Verification items for the finished model (mm, model axes). Face numbers are marked on the shaded views. A direction names the side the tool comes from. Round coordinates to 2 decimals unless told otherwise and drop trailing zeros. Order: outer loops, then holes, each group sorted by start corner. A loop starts at its lowest first (then second) coordinate and runs counter-clockwise, first axis right, second up. Notation, with made-up numbers: M -10.5,17 L 35.5,17 A15 ccw 35.5,24 Z; hole C -11,78 d9. An arc over 180 degrees is marked long. One line per item, written item: value. Start each with the question number.
from build123d import *

# Parameters (mm, degrees)
F0_W     = 63.5000000107
F0_H     = 19.05
F1_DEPTH = 63.5
F0_W_2   = 19.0499999893
F2_DEPTH = 25.4
F3_DEPTH = 15.875
F0_W_3   = 25.4
F0_H_2   = 19.0499999893
F5_R     = 6.35


with BuildPart() as f1:
    # F0 (on Front) → F1 (new body, symmetric)
    with BuildSketch(Plane.XZ):
        with Locations((-9.5249999946, 0)):
            Rectangle(F0_W, F0_H)
    extrude(amount=F1_DEPTH, both=True)

    # F0 (on Front) → F2 (join, symmetric)
    with BuildSketch(Plane.XZ):
        with Locations((31.7500000054, 0)):
            Rectangle(F0_W_2, F0_H)
        with BuildLine():
            Line((22.2250000107, 9.525), (41.275, 9.525))
            Line((41.275, 9.525), (41.275, 27.0002))
            ThreePointArc((41.275, 27.0002), (45.9246798487, 38.2255201513), (57.15, 42.8752))
            Line((57.15, 42.8752), (60.325, 42.8752))
            Line((60.325, 42.8752), (60.325, 61.9251999893))
            Line((60.325, 61.9251999893), (57.1730846286, 61.9251999893))
            Line((57.1730846286, 61.9251999893), (57.15, 61.9251999893))
            ThreePointArc((57.15, 61.9251999893), (32.4542956746, 51.6959043254), (22.2250000107, 27.0002))
            Line((22.2250000107, 27.0002), (22.2250000107, 9.525))
        make_face()
    extrude(amount=F2_DEPTH, both=True)

    # F0 (on Front) → F3 (join)
    with BuildSketch(Plane.XZ):
        with BuildLine():
            Line((-41.275, 9.525), (22.2250000107, 9.525))
            Line((22.2250000107, 9.525), (22.2250000107, 27.0002))
            ThreePointArc((22.2250000107, 27.0002), (32.4542956746, 51.6959043254), (57.15, 61.9251999893))
            add(Edge.make_bspline(
                [(-41.275, 9.525), (-41.275, 48.5757485088), (19.736442486, 61.9251999893), (57.15, 61.9251999893)],
                knots=[0, 0, 0, 0, 111.5045361585, 111.5045361585, 111.5045361585, 111.5045361585], degree=3))
        make_face()
    extrude(amount=F3_DEPTH)

    # F0 (on Front) → F4 (revolve)
    with BuildSketch(Plane.XZ):
        with Locations((73.025, 52.4001999946)):
            Rectangle(F0_W_3, F0_H_2)
    revolve(axis=Axis((60.325, 0, 52.3875), (0, 0, 1)))

    # F5
    f5_edges = [f1.edges().sort_by_distance(p)[0] for p in [
        (-41.275, -63.5, 0),
        (22.225, -63.5, 0),
        (-41.275, 63.5, 0),
        (22.225, 63.5, 0),
    ]]
    fillet(f5_edges, radius=F5_R)


solid = f1.part
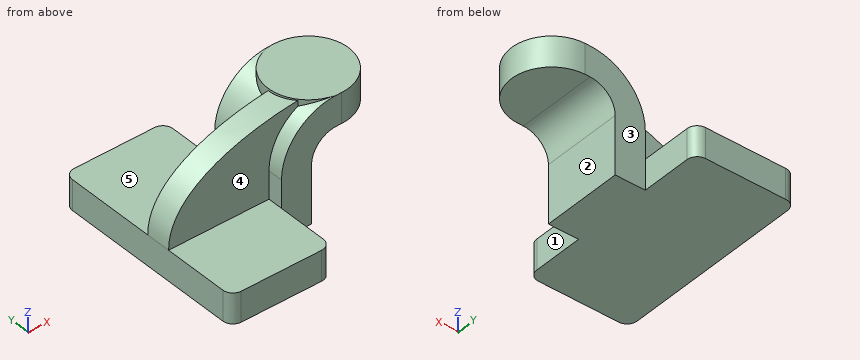
1. Tool access check on the marked faces 1, 2, 3, 4 and 5. Record the directions out of +Z, -Z, +X, -X, +Y, -Y that give a thin tool (end or side, any length) a straight path to the whole face; none if there is none.
2. Section check B-B (x = 64). Record the cut outline in (y, z).
3. Section check A-A (y = 31). Record the cut outline in (x, z) (3 decimals).
4. Scan lines: line 1 along Z through (x, y) = (18, 15) (3 decimals); line 2 along Y through (x, z) = (23.5, -0.5); line 3 along X through (y, z) = (-9, 5.5) (3 decimals). Record each from-to range of solid material in increasing order.
5. Depth check by flat-ended pin: pin 1 (3 mm diameter, centred on x = 1.5, z = 24, fed in from -Y) (3 decimals); pin 2 (8.5 mm diameter, centred on y = 12, z = 19.5, fed in from -X) (3 decimals); pin 3 (15 mm diameter, centred on y = -38.5, z = 4, fed in from +X) (3 decimals). Enter the tip coordinate at first touch or a pass-through.
Geometry check:
1. face 1: +Z, -Z, +X, -Y
1. face 2: -Z, +X, +Y, -Y
1. face 3: +Z, -Z, +X, +Y
1. face 4: +Z, -X, -Y
1. face 5: +Z, -X, +Y
2. outline: M -25.13,42.88 L 25.13,42.88 L 25.13,61.93 L -25.13,61.93 Z
3. outline: M -41.275,-9.525 L 22.225,-9.525 L 22.225,9.525 L -41.275,9.525 Z
4. line 1: z = -9.525 to 9.525
4. line 2: y = -25.4 to 25.4
4. line 3: x = -41.275 to 41.275
5. pin 1: stops at y = -15.875
5. pin 2: stops at x = 22.225
5. pin 3: stops at x = 22.225
